Design review of the part built by this model. Coordinates are the model's own, in mm. Face numbers are marked on the shaded views. A direction names the side the tool comes from. Coordinates: 2 decimals unless noted, no trailing zeros. Write each loop counter-clockwise with the first axis right and the second up, starting at its lowest first coordinate (ties: lowest second). Pieces come first, ordered by that corner, then holes. Notation, with made-up numbers: (-15.75, 51) -> (23.25, 51) arc R27 ccw to (23.25, 79) -> close; hole circle Ø3 at (-12.5, -13). An arc over 180 degrees is marked (long way). One line per question, with ' | ' between items. Start each with the question number.
Q1. For P1, Ø24, axis at y = 29.5, z = 29.5, coming from the -X side; P2, Ø3, axis at y = 6.5, z = 62, coming from the +X side; P3, Ø24, axis at x = 58, y = -29, coming from the +Z side; P4, Ø5, axis at x = 30, z = 12, coming from the -Y side, all flat-tipped, find the tip position at first contact; note any pin that passes through.
Q2. Draft analysis for pull direction Y (two halves, no side actions). For the marked faces 4, 5 and 6, state which applies: pulls with the +Y half, pulls with the -Y half, needs draft (parallel to the pull), parting line crosses it, or undercut.
Q3. Add section D-D on x = 18.5. State the section outline as (y, z) points.
Q4. Add section B-B on y = 22.5. State the section outline as (x, z) points.
Q5. For the marked faces 1, 2 and 3, list the 3-axis set-ups (+Z, -Z, +X, -X, +Y, -Y) from which the entire face can be reached by the end or side of a thin tool; tool diameter is ignored.
Q6. Add section C-C on y = -25. State the section outline as (x, z) points, and give its area (3 significant figures).
Q7. Add section A-A on x = -52.5. State the section outline as (y, z) points, and give its area (3 significant figures).
Q8. Wall thickness on probe 1 along Y at (x, z) = (52, -4); probe 2 along Z at (x, y) = (-61, 17.5); probe 3 along X at (y, z) = (-37, 13.5): over which ranges is each line inside the solid? List them lowest first.
from build123d import *

# Parameters (mm, degrees)
SKETCH1_W           = 75
SKETCH1_H           = 90
BOSS_EXTRUDE1_DEPTH = 10
SKETCH2_W           = 75
SKETCH2_H           = 40
BOSS_EXTRUDE2_DEPTH = 45
SKETCH5_W           = 10
SKETCH5_H           = 90
BOSS_EXTRUDE3_DEPTH = 10
SKETCH7_W           = 10
SKETCH7_H           = 90
BOSS_EXTRUDE4_DEPTH = 30
SKETCH14_R          = 20
BOSS_EXTRUDE6_DEPTH = 75
SKETCH15_R          = 10
CUT_EXTRUDE3_DEPTH  = 75
SKETCH16_R          = 6
CUT_EXTRUDE4_DEPTH  = 75
RIB16_REACH         = 112.482
SKETCH24_WALL_W     = 290.231918176
SKETCH24_WALL_H     = 10
RIB17_REACH         = 115.975
SKETCH25_WALL_W     = 261.572332424
SKETCH25_WALL_H     = 10
RIB18_REACH         = 115.975
SKETCH26_WALL_W     = 261.572332424
SKETCH26_WALL_H     = 10


with BuildPart() as part:
    # Sketch1 → Boss-Extrude1 (new body)
    with BuildSketch(Plane.XY):
        Rectangle(SKETCH1_W, SKETCH1_H)
    extrude(amount=BOSS_EXTRUDE1_DEPTH)

    # Sketch2 → Boss-Extrude2 (add)
    with BuildSketch(Plane.XY.offset(10)):
        with Locations((0, 25)):
            Rectangle(SKETCH2_W, SKETCH2_H)
    extrude(amount=BOSS_EXTRUDE2_DEPTH)

    # Sketch5 → Boss-Extrude3 (add)
    with BuildSketch(Plane(origin=(0, 0, 0), x_dir=(-1, 0, 0), z_dir=(0, 0, -1))):
        with Locations((-32.5, 0)):
            Rectangle(SKETCH5_W, SKETCH5_H)
        with Locations((32.5, 0)):
            Rectangle(SKETCH5_W, SKETCH5_H)
    boss_extrude3 = extrude(amount=BOSS_EXTRUDE3_DEPTH)

    # Sketch7 → Boss-Extrude4 (add)
    with BuildSketch(Plane(origin=(37.5, 0, 0), x_dir=(0, 0, -1), z_dir=(1, 0, 0))):
        with Locations((5, 0)):
            Rectangle(SKETCH7_W, SKETCH7_H)
    boss_extrude4 = extrude(amount=BOSS_EXTRUDE4_DEPTH)

    # Mirror1: Boss-Extrude3, Boss-Extrude4 across plane
    add(boss_extrude3.mirror(Plane(origin=(0, 0, 0), x_dir=(0, 0, 1), z_dir=(1, 0, 0))))
    add(boss_extrude4.mirror(Plane(origin=(0, 0, 0), x_dir=(0, 0, 1), z_dir=(1, 0, 0))))

    # Sketch14 → Boss-Extrude6 (add)
    with BuildSketch(Plane.ZY.offset(37.5)):
        with Locations((55, 25)):
            Circle(SKETCH14_R)
    extrude(amount=-BOSS_EXTRUDE6_DEPTH)

    # Sketch15 → Cut-Extrude3 (cut)
    with BuildSketch(Plane.ZY.offset(37.5)):
        with Locations((45, 25)):
            Circle(SKETCH15_R)
    extrude(amount=-CUT_EXTRUDE3_DEPTH, mode=Mode.SUBTRACT)

    # Sketch16 → Cut-Extrude4 (cut)
    with BuildSketch(Plane.XY):
        with Locations((-52.5, 25)):
            Circle(SKETCH16_R)
        with Locations((52.5, 25)):
            Circle(SKETCH16_R)
        with Locations(Location((52.5, -25, 0), (0, 0, 180))):
            Circle(SKETCH16_R)
        with Locations((-52.5, -25)):
            Circle(SKETCH16_R)
    extrude(amount=-CUT_EXTRUDE4_DEPTH, mode=Mode.SUBTRACT)

    # Sketch24 wall → Rib16 (add, up to next)
    with BuildSketch(Plane(origin=(0, -20, 32.5), x_dir=(0, 0.743294146247, 0.668964731622), z_dir=(0, 0.668964731622, -0.743294146247)), mode=Mode.PRIVATE) as rib16_sk1:
        Rectangle(SKETCH24_WALL_W, SKETCH24_WALL_H)
    rib16_tool1 = extrude(rib16_sk1.sketch, amount=RIB16_REACH, mode=Mode.PRIVATE) - part.part
    add(rib16_tool1.solids().sort_by_distance((0, -20, 32.5))[0])

    # Sketch25 wall → Rib17 (add, up to next)
    with BuildSketch(Plane(origin=(52.5, -8, 5), x_dir=(-0.948683298051, 0, 0.316227766017), z_dir=(-0.316227766017, 0, -0.948683298051)), mode=Mode.PRIVATE) as rib17_sk1:
        Rectangle(SKETCH25_WALL_W, SKETCH25_WALL_H)
    rib17_tool1 = extrude(rib17_sk1.sketch, amount=RIB17_REACH, mode=Mode.PRIVATE) - part.part
    add(rib17_tool1.solids().sort_by_distance((52.5, -8, 5))[0])

    # Sketch26 wall → Rib18 (add, up to next)
    with BuildSketch(Plane(origin=(-52.5, -8, 5), x_dir=(0.948683298051, 0, 0.316227766017), z_dir=(-0.316227766017, 0, 0.948683298051)), mode=Mode.PRIVATE) as rib18_sk1:
        Rectangle(SKETCH26_WALL_W, SKETCH26_WALL_H)
    rib18_tool1 = extrude(rib18_sk1.sketch, amount=-RIB18_REACH, mode=Mode.PRIVATE) - part.part
    add(rib18_tool1.solids().sort_by_distance((-52.5, -8, 5))[0])


solid = part.part
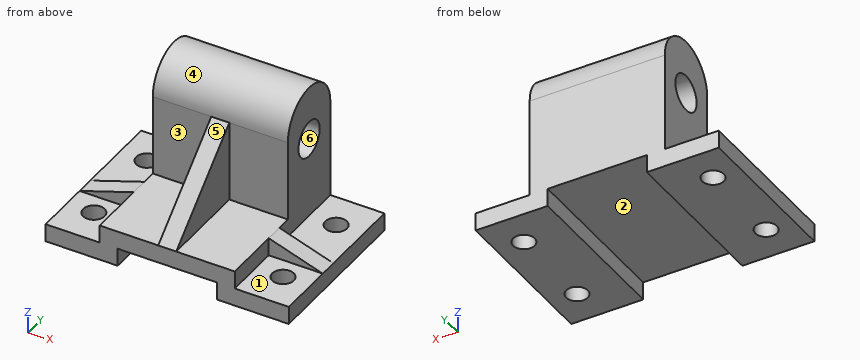
Output values:
1) P1: stops at x = -37.5 | P2: stops at x = 37.5 | P3: stops at z = 0 | P4: stops at y = -45
2) face 4: parting line crosses it | face 5: pulls with the -Y half | face 6: undercut
3) outline: (-45, 0) -> (45, 0) -> (45, 55) arc R20 ccw to (5, 55) -> (5, 10) -> (-45, 10) -> close; hole circle Ø20 at (25, 45)
4) outline: (-67.5, -10) -> (-57.95, -10) -> (-57.95, 0) -> (-67.5, 0) -> close; (-47.05, -10) -> (-27.5, -10) -> (-27.5, 0) -> (27.5, 0) -> (27.5, -10) -> (47.05, -10) -> (47.05, 0) -> (37.5, 0) -> (37.5, 35.32) -> (-37.5, 35.32) -> (-37.5, 0) -> (-47.05, 0) -> close; (-37.5, 54.68) -> (37.5, 54.68) -> (37.5, 74.84) -> (-37.5, 74.84) -> close; (57.95, -10) -> (67.5, -10) -> (67.5, 0) -> (57.95, 0) -> close
5) face 1: +Z, +X, -Y | face 2: -Z, +Y, -Y | face 3: +Z, -X, -Y
6) outline: (-67.5, -10) -> (-58.5, -10) -> (-58.5, 0) -> (-67.5, 0) -> close; (-46.5, -10) -> (-27.5, -10) -> (-27.5, 0) -> (27.5, 0) -> (27.5, -10) -> (46.5, -10) -> (46.5, 0) -> (37.5, 0) -> (37.5, 10) -> (5, 10) -> (5, 28) -> (-5, 28) -> (-5, 10) -> (-37.5, 10) -> (-37.5, 0) -> (-46.5, 0) -> close; (58.5, -10) -> (67.5, -10) -> (67.5, 0) -> (58.5, 0) -> close | area: 1,490 mm2
7) outline: (-45, -10) -> (-31, -10) -> (-31, 0) -> (-45, 0) -> close; (-19, -10) -> (19, -10) -> (19, 0) -> (-3, 0) -> (-3, 5) -> (-13, 5) -> (-13, 0) -> (-19, 0) -> close; (31, -10) -> (45, -10) -> (45, 0) -> (31, 0) -> close | area: 710 mm2
8) probe 1: y = -45 to -30.98, -19.02 to 19.02, 30.98 to 45 | probe 2: z = -10 to 0 | probe 3: x = -5 to 5
